Geometry check sheet. Reference: the model listing, model coordinates, mm. A direction names the side the tool comes from. Round coordinates to 2 decimals unless told otherwise and drop trailing zeros. Write each loop counter-clockwise with the first axis right and the second up, starting at its lowest first coordinate (ties: lowest second). Pieces come first, ordered by that corner, then holes.
Item 1: Scan lines: probe 1 along Z at (x, y) = (0, 14); probe 2 along Z at (x, y) = (53, -18); probe 3 along Y at (x, z) = (71, 13). Record each from-to range of solid material in increasing order.
Item 2: Depth check by flat-ended pin: P1, Ø23, axis at x = 0, z = 75, coming from the +Y side; P2, Ø1.5, axis at y = 9, z = 81, coming from the +X side; P3, Ø12, axis at x = 38.5, y = -16.5, coming from the +Z side. Enter the tip coordinate at first touch or a pass-through.
Item 3: Cross-section at B-B (z = 56). Enter the section's corners in (x, y), then the cut area to 3 significant figures.
Item 4: Draft check along Z on faces 1 (the face through (-1.302, 12.923, 84.915)), 2 (the face through (0, -7.5, 63)), 3 (the face through (0, -23, 50)), 4 (the face through (-1.302, -13.077, 84.915)). Enter one of: pulls with the +Z half, pulls with the -Z half, needs draft (parallel to the pull), parting line crosses it, or undercut.
Item 5: Access from +Z, -Z, +X, -X, +Y, -Y to the whole of each face (thin tool, end or side, straight path). Record for faces 5 (the face through (0.554, 29.995, 49.3)), 6 (the face through (39.779, -22.095, 12.325)), 7 (the face through (10.2, -18.5, 75.4)), 8 (the face through (-11, 18.5, 75)).
Item 6: Cross-section at D-D (x = -71). Enter the section's corners in (y, z), then the cut area to 3 significant figures.
Item 7: Cross-section at A-A (x = 0). Enter the section's corners in (y, z).
Item 8: Cross-section at C-C (y = -2). Enter the section's corners in (x, z).
from build123d import *

# Parameters (mm, degrees)
F0_R     = 7.5
F1_DEPTH = 25
F2_DEPTH = 100
F3_W     = 80
F3_H     = 15
F4_DEPTH = 75
F5_W     = 130
F5_H     = 70
F5_W_2   = 100
F5_H_2   = 37
F6_DEPTH = 50
F7_R     = 10
F8_DEPTH = 25


with BuildPart() as f1:
    # F0 (on Top) → F1 (new body)
    with BuildSketch(Plane.XY):
        with BuildLine():
            ThreePointArc((-74.1690140845, -14.6614238644), (-61.5802126157, -11.6733716481), (-56, 0))
            ThreePointArc((-56, 0), (-61.5802126157, 11.6733716481), (-74.1690140845, 14.6614238644))
            ThreePointArc((-74.1690140845, 14.6614238644), (-86, 0), (-74.1690140845, -14.6614238644))
        make_face()
        with Locations((-71, 0)):
            Circle(F0_R, mode=Mode.SUBTRACT)
        with BuildLine():
            ThreePointArc((-74.1690140845, 14.6614238644), (-61.5802126157, 11.6733716481), (-56, 0))
            ThreePointArc((-56, 0), (-61.5802126157, -11.6733716481), (-74.1690140845, -14.6614238644))
            Line((-74.1690140845, -14.6614238644), (-6.338028169, -29.3228477288))
            ThreePointArc((-6.338028169, -29.3228477288), (-30, 0), (-6.338028169, 29.3228477288))
            Line((-6.338028169, 29.3228477288), (-74.1690140845, 14.6614238644))
        make_face()
        with BuildLine():
            ThreePointArc((6.338028169, 29.3228477288), (0, 30), (-6.338028169, 29.3228477288))
            ThreePointArc((-6.338028169, 29.3228477288), (-30, 0), (-6.338028169, -29.3228477288))
            ThreePointArc((-6.338028169, -29.3228477288), (0, -30), (6.338028169, -29.3228477288))
            ThreePointArc((6.338028169, -29.3228477288), (23.3467432961, -18.8395747687), (30, 0))
            ThreePointArc((30, 0), (23.3467432961, 18.8395747687), (6.338028169, 29.3228477288))
        make_face()
        with BuildLine():
            Line((74.1690140845, 14.6614238644), (6.338028169, 29.3228477288))
            ThreePointArc((6.338028169, 29.3228477288), (23.3467432961, 18.8395747687), (30, 0))
            ThreePointArc((30, 0), (23.3467432961, -18.8395747687), (6.338028169, -29.3228477288))
            Line((6.338028169, -29.3228477288), (74.1690140845, -14.6614238644))
            ThreePointArc((74.1690140845, -14.6614238644), (56, 0), (74.1690140845, 14.6614238644))
        make_face()
        with BuildLine():
            ThreePointArc((86, 0), (82.6733716481, 9.4197873843), (74.1690140845, 14.6614238644))
            ThreePointArc((74.1690140845, 14.6614238644), (56, 0), (74.1690140845, -14.6614238644))
            ThreePointArc((74.1690140845, -14.6614238644), (82.6733716481, -9.4197873843), (86, 0))
        make_face()
        with Locations((71, 0)):
            Circle(F0_R, mode=Mode.SUBTRACT)
    extrude(amount=F1_DEPTH)

    # F0 (on Top) → F2 (join)
    with BuildSketch(Plane.XY):
        with BuildLine():
            ThreePointArc((6.338028169, 29.3228477288), (0, 30), (-6.338028169, 29.3228477288))
            ThreePointArc((-6.338028169, 29.3228477288), (-30, 0), (-6.338028169, -29.3228477288))
            ThreePointArc((-6.338028169, -29.3228477288), (0, -30), (6.338028169, -29.3228477288))
            ThreePointArc((6.338028169, -29.3228477288), (23.3467432961, -18.8395747687), (30, 0))
            ThreePointArc((30, 0), (23.3467432961, 18.8395747687), (6.338028169, 29.3228477288))
        make_face()
    extrude(amount=F2_DEPTH)

    # F3 (on face) → F4 (cut, through all)
    with BuildSketch(Plane.XY.offset(100)):
        Rectangle(F3_W, F3_H)
    extrude(amount=-F4_DEPTH, mode=Mode.SUBTRACT)

    # F5 (on face) → F6 (cut)
    with BuildSketch(Plane.XY.offset(100)):
        Rectangle(F5_W, F5_H)
        Rectangle(F5_W_2, F5_H_2, mode=Mode.SUBTRACT)
    extrude(amount=-F6_DEPTH, mode=Mode.SUBTRACT)

    # F7 (on Front) → F8 (cut, symmetric)
    with BuildSketch(Plane.XZ):
        with Locations((0, 75)):
            Circle(F7_R)
    extrude(amount=F8_DEPTH, both=True, mode=Mode.SUBTRACT)


solid = f1.part
Resolved:
1. probe 1: z = 0 to 65, 85 to 100
1. probe 2: z = 0 to 25
1. probe 3: y = -15.35 to -7.5, 7.5 to 15.35
2. P1: stops at y = 18.5
2. P2: stops at x = 28.84
2. P3: stops at z = 25
3. outline: (-29.05, -7.5) arc R30 ccw to (-23.62, -18.5) - (23.62, -18.5) arc R30 ccw to (29.05, -7.5) - close; (-29.05, 7.5) - (29.05, 7.5) arc R30 ccw to (23.62, 18.5) - (-23.62, 18.5) arc R30 ccw to start
3. area: 1,180 mm2
4. face 1: undercut
4. face 2: needs draft
4. face 3: pulls with the +Z half
4. face 4: undercut
5. face 5: +Z, +Y
5. face 6: +Z, -Z, +X, -Y
5. face 7: +Z, +X, -X, -Y
5. face 8: +Z, +X, -X, +Y
6. outline: (-15.35, 0) - (-7.5, 0) - (-7.5, 25) - (-15.35, 25) - close; (7.5, 0) - (15.35, 0) - (15.35, 25) - (7.5, 25) - close
6. area: 392 mm2
7. outline: (-30, 0) - (30, 0) - (30, 50) - (18.5, 50) - (18.5, 65) - (7.5, 65) - (7.5, 25) - (-7.5, 25) - (-7.5, 65) - (-18.5, 65) - (-18.5, 50) - (-30, 50) - close; (-18.5, 85) - (-7.5, 85) - (-7.5, 100) - (-18.5, 100) - close; (7.5, 85) - (18.5, 85) - (18.5, 100) - (7.5, 100) - close
8. outline: (-85.87, 0) - (-78.23, 0) - (-78.23, 25) - (-85.87, 25) - close; (-63.77, 0) - (63.77, 0) - (63.77, 25) - (-63.77, 25) - close; (78.23, 0) - (85.87, 0) - (85.87, 25) - (78.23, 25) - close
